Part model, mm, in its own coordinate system. A direction names the side the tool comes from. Round coordinates to 2 decimals unless told otherwise and drop trailing zeros. Order: outer loops, then holes, each group sorted by start corner. A loop starts at its lowest first (then second) coordinate and runs counter-clockwise, first axis right, second up. Notation, with made-up numbers: M 8,28.5 L 35,28.5 A32 ccw 35,64.5 Z; hole C 50.25,75.5 d4. An arc over 180 degrees is marked long. One line per question, with ' | ' between items.
from build123d import *

# Parameters (mm, degrees)
SKETCH1_W               = 139.7
SKETCH1_H               = 139.7
BOSS_EXTRUDE1_DEPTH     = 139.7
FILLET1_R               = 7.62
FILLET2_R               = 7.62
BOSS_EXTRUDE3_REACH     = 210.999
CUT_EXTRUDE2_DEPTH      = 209.804
SKETCH9_R               = 45.72
CUT_EXTRUDE3_DEPTH      = 209.804
BOSS_EXTRUDE4_REACH     = 231.134
CUT_EXTRUDE4_REACH      = 231.134
CUT_EXTRUDE4_END_RADIUS = 45.72
SKETCH11_R              = 16.51


with BuildPart() as part:
    # Sketch1 → Boss-Extrude1 (new body)
    with BuildSketch(Plane.XY):
        Rectangle(SKETCH1_W, SKETCH1_H)
    extrude(amount=BOSS_EXTRUDE1_DEPTH)

    # Fillet1
    fillet1_edges = [part.edges().sort_by_distance(p)[0] for p in [
        (-69.85, 69.85, 69.85),
    ]]
    fillet(fillet1_edges, radius=FILLET1_R)

    # Fillet2
    fillet2_edges = [part.edges().sort_by_distance(p)[0] for p in [
        (69.85, -69.85, 69.85),
        (-69.85, -69.85, 69.85),
        (69.85, 69.85, 69.85),
    ]]
    fillet(fillet2_edges, radius=FILLET2_R)

    # Sketch6 → Boss-Extrude3 (add, up to next)
    with BuildSketch(Plane(origin=(32.818764781, 46.870053506, 0), x_dir=(0, 0, 1), z_dir=(0.5735764363510473, 0.819152044288991, 0)), mode=Mode.PRIVATE) as boss_extrude3_sk1:
        with BuildLine():
            Line((38.072922524, -40.064314079), (101.627077476, -40.064314079))
            ThreePointArc((101.627077476, -40.064314079), (121.947077476, -60.384314079), (101.627077476, -80.704314079))
            Line((101.627077476, -80.704314079), (38.072922524, -80.704314079))
            ThreePointArc((38.072922524, -80.704314079), (17.752922524, -60.384314079), (38.072922524, -40.064314079))
        make_face()
    boss_extrude3_tool1 = extrude(boss_extrude3_sk1.sketch, amount=-BOSS_EXTRUDE3_REACH, mode=Mode.PRIVATE) - part.part
    add(boss_extrude3_tool1.solids().sort_by_distance((-16.64517, 81.505073, 69.85))[0])

    # Sketch8 → Cut-Extrude2 (cut)
    with BuildSketch(Plane(origin=(32.818764781, 46.870053506, 0), x_dir=(0.819152044288991, -0.5735764363510474, 0), z_dir=(0.5735764363510474, 0.819152044288991, 0))):
        with BuildLine():
            Line((-70.544314079, -101.627077476), (-70.544314079, -38.072922524))
            ThreePointArc((-70.544314079, -38.072922524), (-60.384314079, -27.912922524), (-50.224314079, -38.072922524))
            Line((-50.224314079, -38.072922524), (-50.224314079, -101.627077476))
            ThreePointArc((-50.224314079, -101.627077476), (-60.384314079, -111.787077476), (-70.544314079, -101.627077476))
        make_face()
    extrude(amount=-CUT_EXTRUDE2_DEPTH, mode=Mode.SUBTRACT)

    # Sketch9 → Cut-Extrude3 (cut)
    with BuildSketch(Plane.XY.offset(139.7)):
        Circle(SKETCH9_R)
    extrude(amount=-CUT_EXTRUDE3_DEPTH, mode=Mode.SUBTRACT)

    # Boss-Extrude4: up to this face of the body (flat: up to its plane)
    boss_extrude4_end = Plane(part.part.faces().sort_by_distance((69.85, 0, 69.85))[0])
    # Sketch10 → Boss-Extrude4 (add, up to the picked face)
    with BuildSketch(Plane(origin=(52.3875, 0, -30.245937227), x_dir=(0, 1, 0), z_dir=(0.866025403784438, 0, -0.5000000000000009)), mode=Mode.PRIVATE) as boss_extrude4_sk1:
        with BuildLine():
            Line((-50.8, 34.925), (50.8, 34.925))
            ThreePointArc((50.8, 34.925), (0, 85.725), (-50.8, 34.925))
        make_face()
    boss_extrude4_tool1 = split(extrude(boss_extrude4_sk1.sketch, amount=-BOSS_EXTRUDE4_REACH, mode=Mode.PRIVATE), bisect_by=boss_extrude4_end, keep=Keep.BOTH, mode=Mode.PRIVATE)
    boss_extrude4 = boss_extrude4_tool1.solids().sort_by(Axis((80.630095, 0, 18.671672), (-0.866025403784438, 0, 0.5000000000000009)))[0]
    add(boss_extrude4)

    # Cut-Extrude4: up to this cylinder (the profile starts outside it)
    cut_extrude4_end = Plane(origin=(0, 0, 21.117163), z_dir=(0, 0, 1)) * Cylinder(CUT_EXTRUDE4_END_RADIUS, 554.708, mode=Mode.PRIVATE)
    # Sketch11 → Cut-Extrude4 (cut, up to the surface)
    with BuildSketch(Plane(origin=(52.3875, 0, -30.245937227), x_dir=(-0.5000000000000012, 0, -0.866025403784438), z_dir=(0.8660254037844379, 0, -0.5000000000000011)), mode=Mode.PRIVATE) as cut_extrude4_sk1:
        with Locations((-59.309, 0)):
            Circle(SKETCH11_R)
    cut_extrude4_tool1 = extrude(cut_extrude4_sk1.sketch, amount=-CUT_EXTRUDE4_REACH, mode=Mode.PRIVATE) - cut_extrude4_end
    cut_extrude4 = cut_extrude4_tool1.solids().sort_by_distance((82.042, 0, 21.117163))[0]
    add(cut_extrude4, mode=Mode.SUBTRACT)

    # Mirror1: Boss-Extrude4, Cut-Extrude4 across plane
    add(boss_extrude4.mirror(Plane.XY.offset(69.85)))
    add(cut_extrude4.mirror(Plane.XY.offset(69.85)), mode=Mode.SUBTRACT)


solid = part.part
1) Saw through at A-A (x = 22). List the corners of the cut face in (y, z).
The answers:
outline: M -69.85,0 L -40.08,0 L -40.08,139.7 L -69.85,139.7 Z; M 40.08,0 L 69.85,0 L 69.85,139.7 L 40.08,139.7 Z
2) Two-plate mould, pull along Y, no slides. Class faces 1 (the face through (-38.656, 32.358, 69.405)), 2 (the face through (-1, -69.85, 69)), 3 (the face through (-1, 48, 0)): released by +Y, released by -Y, zero draft, split by the parting line, or undercut.
The answers:
face 1: undercut | face 2: released by -Y | face 3: zero draft
3) Which spindle directions (+Z, -Z, +X, -X, +Y, -Y) get a long thin tool onto all of the face, cutting with end or side? Do faces 4 (the face through (85.544, 1.117, 49.584)), 5 (the face through (74.26, -12, 132.06)). Say none if no direction does.
The answers:
face 4: +X | face 5: +Z, +X, +Y, -Y
4) Saw through at B-B (x = -42.5). Give the number of separate pieces and of enclosed holes in the cut face, plus the area to 3 significant figures.
The answers:
separate pieces: 2 | enclosed holes: 1 | area: 12,800 mm²
5) Saw through at C-C (y = -56). List the corners of the cut face in (x, z), plus the area to 3 significant figures.
The answers:
outline: M -69.85,0 L 69.85,0 L 69.85,139.7 L -69.85,139.7 Z | area: 19,500 mm²
6) Probe line 1 (Y direction, x = 0, z = 103); line 2 (Z direction, x = 49, y = 1); line 3 (Y direction, x = 36.5, z = 27). List the from-to ranges inside material, lowest first. Write a range as [from, to].
The answers:
line 1: y = [-69.85, -45.72], [45.72, 69.85] | line 2: z = [0, 21.16], [59.22, 80.48], [118.54, 139.7] | line 3: y = [-69.85, -27.53], [27.53, 69.85]
7) Drop flat-ended pins along their axis: pin 1 (8 mm diameter, centred on x = -44, z = 48, fed in from +Y); pin 2 (8 mm diameter, centred on y = 10, z = 53.5, fed in from -X); pin 3 (5 mm diameter, centred on x = 33, z = 112.5, fed in from +Y); pin 4 (5 mm diameter, centred on x = -28, y = -43.5, fed in from -Z). Give the stop position or say it passes through.
The answers:
pin 1: stops at y = 83.58 | pin 2: stops at x = -57.11 | pin 3: stops at y = 69.85 | pin 4: stops at z = 0
